```python
from build123d import *

# Parameters (mm, degrees)
F0_R     = 3.175
F1_DEPTH = 6.35


# Not quite as in the source:
# - ends of sketch curves that miss each other by under 0.0002 mm in the source are joined


with BuildPart() as f1:
    # F0 (on Right) → F1 (new body)
    with BuildSketch(Plane.YZ):
        with BuildLine():
            Line((-88.9, -53.975), (-88.9, -130.175))
            Line((-88.9, -130.175), (-98.425, -130.175))
            Line((-98.425, -130.175), (-98.425, -139.7))
            Line((-98.425, -139.7), (98.425, -139.7))
            Line((98.425, -139.7), (98.425, -130.175))
            Line((98.425, -130.175), (88.9, -130.175))
            Line((88.9, -130.175), (88.9, -53.975))
            Line((88.9, -53.975), (82.55, -53.975))
            Line((82.55, -53.975), (82.55, 28.575))
            Line((82.55, 28.575), (76.2, 28.575))
            Line((76.2, 28.575), (76.2, 34.925))
            Line((76.2, 34.925), (76.2, 131.7625))
            ThreePointArc((76.2, 131.7625), (68.2625, 139.7), (60.325, 131.7625))
            Line((60.325, 131.7625), (60.325, 114.3))
            ThreePointArc((60.325, 114.3), (42.8625, 107.8115954), (25.3999938624, 114.299992881))
            ThreePointArc((25.3999938624, 114.299992881), (0, 139.7), (-25.4, 114.3))
            Line((-25.4, 114.3), (-76.2, 41.275))
            Line((-76.2, 41.275), (-76.2, 28.575))
            Line((-76.2, 28.575), (-82.55, 28.575))
            Line((-82.55, 28.575), (-82.55, -53.975))
            Line((-82.55, -53.975), (-88.9, -53.975))
        make_face()
        with Locations((0, 114.3)):
            Circle(F0_R, mode=Mode.SUBTRACT)
    extrude(amount=F1_DEPTH)


solid = f1.part
```
For this review, take the finished solid that the model builds, in its own axes (mm). A direction names the side the tool comes from. Round coordinates to 2 decimals unless told otherwise and drop trailing zeros. Write each loop counter-clockwise with the first axis right and the second up, starting at its lowest first coordinate (ties: lowest second). Pieces come first, ordered by that corner, then holes. Notation, with made-up numbers: M -19.5,41 L -11.5,41 A6 ccw -11.5,52 Z; hole C 21,-31 d8. An arc over 180 degrees is marked long. One line per item, written item: value. Start each with the question number.
(1) We need section A-A (y = 0). Give the boundary of the cut face in (x, z) (3 decimals), and give its area (3 significant figures).
(2) Machinability: for faces 1 (the flat face through (3, -79, 28.575)), 2 (the flat face through (3, 98.425, -135)), 3 (the flat face through (3, 94, -130.175)), which of the approach directions +Z, -Z, +X, -X, +Y, -Y give a long, thin tool a straight path to every point of the face, cutting with its end or side? Answer none if there is none.
(3) The part is to be moulded in two halves that separate along Y. For faces 4 (the flat face through (3, 60.325, 123)), 5 (the flat face through (3, -86, -53.975)), 6 (the flat face through (3, -88.9, -92)), say which applies: released by +Y, released by -Y, zero draft, split by the parting line, or undercut.
(4) Insertion check: pin 1 (3 mm diameter, centred on x = 4.5, z = 63, fed in from +Y); pin 2 (3 mm diameter, centred on x = 3.5, y = 87, fed in from +Z) (3 decimals); pin 3 (3 mm diameter, centred on x = 4, y = -80.5, fed in from +Z) (3 decimals). Each pin has a flat end and moves straight along its axis. Give the tip position at first contact, or say it passes through.
(5) We need section D-D (y = 79.5). Give the boundary of the cut face in (x, z) (3 decimals).
(6) Wall thickness on line 1 (Z direction, x = 3, y = 0) (3 decimals); line 2 (Z direction, x = 0.75, y = -88) (3 decimals); line 3 (Y direction, x = 2, z = 39.5): over which ranges is each line inside the solid? List them lowest first.
(7) We need section C-C (z = -80.5). Give the boundary of the cut face in (x, y).
Result:
1. outline: M 0,-139.7 L 6.35,-139.7 L 6.35,111.125 L 0,111.125 Z; M 0,117.475 L 6.35,117.475 L 6.35,139.7 L 0,139.7 Z
1. area: 1,730 mm²
2. face 1: +Z, +X, -X, -Y
2. face 2: +Z, -Z, +X, -X, +Y
2. face 3: +Z, +X, -X, +Y
3. face 4: undercut
3. face 5: zero draft
3. face 6: released by -Y
4. pin 1: y = 76.2
4. pin 2: z = -53.975
4. pin 3: z = 28.575
5. outline: M 0,-139.7 L 6.35,-139.7 L 6.35,28.575 L 0,28.575 Z
6. line 1: -139.7 to 111.125, 117.475 to 139.7
6. line 2: -139.7 to -53.975
6. line 3: -76.2 to 76.2
7. outline: M 0,-88.9 L 6.35,-88.9 L 6.35,88.9 L 0,88.9 Z
